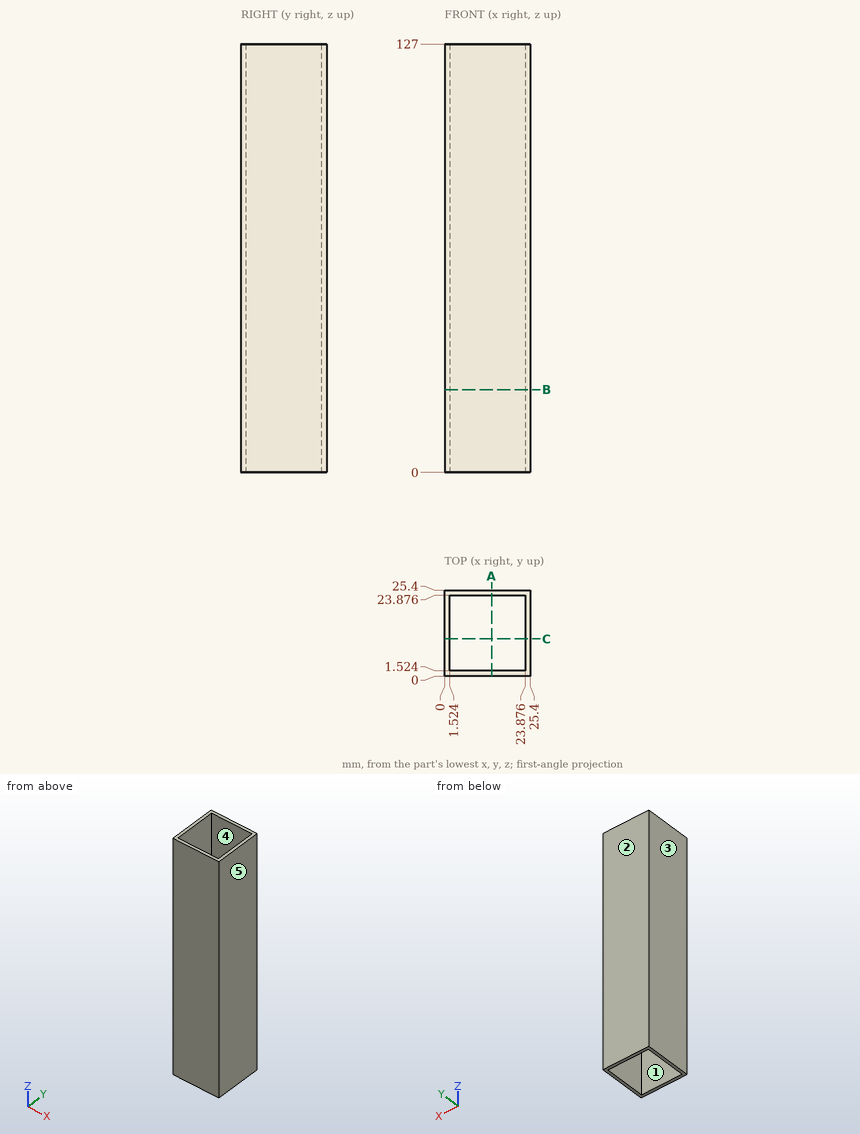
Here's the drawing with two shaded views (mm, measured from the low corner). I have some questions. A direction names the side the tool comes from. Coordinates: 2 decimals unless noted, no trailing zeros. Write each loop counter-clockwise with the first axis right and the second up, starting at its lowest first coordinate (ties: lowest second). Pieces come first, ordered by that corner, then holes. Notation, with made-up numbers: M 58,10.5 L 69,10.5 A9 cw 69,15.5 Z; hole C -26.75,66 d5. An arc over 180 degrees is marked long. Answer as CSV lines item,"result". Start each with the question number.
1) For the marked faces 4 and 5, which set-ups out of +Z, -Z, +X, -X, +Y, -Y let a thin tool reach every point of the face, with its end or its side?
2) We'd pull the mould along Y, two halves only. Please class the marked faces 1, 2 and 3: +Y half, -Y half, draft (parallel to the pull), parting line (faces both ways), or undercut.
3) I want a section at A-A, the plane x = 14. Please give me the cut outline in (y, z).
4) Please list where this line runs through material, in increasing order: line 1 (Y direction, x = 12.5, z = 10.5). Write a range as from..to.
5) I want a section at B-B, the plane z = 24.5. Please give me the cut outline in (x, y).
Data:
1,face 4,"+Z, -Z"
1,face 5,"+Z, -Z, +X, +Y, -Y"
2,face 1,"undercut"
2,face 2,"+Y half"
2,face 3,"draft"
3,outline,"M 0,0 L 1.52,0 L 1.52,127 L 0,127 Z; M 23.88,0 L 25.4,0 L 25.4,127 L 23.88,127 Z"
4,line 1,"y = 0..1.52, 23.88..25.4"
5,outline,"M 0,0 L 25.4,0 L 25.4,25.4 L 0,25.4 Z; hole M 1.52,1.52 L 23.88,1.52 L 23.88,23.88 L 1.52,23.88 Z"
